from build123d import *

# Parameters (mm, degrees)
SKETCH1_W                = 84.074
SKETCH1_H                = 77.724
BOSS_EXTRUDE1_DEPTH      = 5.08
BOSS_EXTRUDE1_DEPTH_BACK = 5.08
SKETCH2_W                = 84.074
SKETCH2_H                = 77.724
BOSS_EXTRUDE2_DEPTH      = 5.08
BOSS_EXTRUDE2_DEPTH_BACK = 10.16
SKETCH3_W                = 53.086
SKETCH3_H                = 5.08
CUT_EXTRUDE1_DEPTH       = 6.08
CUT_EXTRUDE1_DEPTH_BACK  = 11.16
SKETCH4_W                = 75.946
SKETCH4_H                = 5.08
CUT_EXTRUDE2_DEPTH       = 6.08
CUT_EXTRUDE2_DEPTH_BACK  = 11.16
SKETCH5_W                = 75.946
SKETCH5_H                = 7.62
BOSS_EXTRUDE3_DEPTH      = 5.08
BOSS_EXTRUDE3_DEPTH_BACK = 10.16
SKETCH10_R               = 5.08
CUT_EXTRUDE4_DEPTH       = 6.08
CUT_EXTRUDE4_DEPTH_BACK  = 11.16
FILLET1_R                = 10.16
SKETCH14_W               = 63.5
SKETCH14_H               = 3.429
BOSS_EXTRUDE7_DEPTH      = 3.048
CUT_EXTRUDE6_START       = -16.24
SKETCH15_R               = 2.54
SKETCH15_W               = 7.62
SKETCH15_H               = 3.048
CUT_EXTRUDE6_DEPTH       = 20.288
SKETCH7_W                = 34.036
SKETCH7_H                = 5.08
CUT_EXTRUDE7_DEPTH       = 5.064


with BuildPart() as part:
    # Sketch1 → Boss-Extrude1 (new body, two sides)
    with BuildSketch(Plane(origin=(0, 0, 0), x_dir=(1, 0, 0), z_dir=(0, 1, 0))) as boss_extrude1_sk:
        Rectangle(SKETCH1_W, SKETCH1_H)
    extrude(amount=BOSS_EXTRUDE1_DEPTH)
    extrude(boss_extrude1_sk.sketch, amount=-BOSS_EXTRUDE1_DEPTH_BACK)

    # Sketch2 → Boss-Extrude2 (add, two sides)
    with BuildSketch(Plane(origin=(0, 5.08, 0), x_dir=(1, 0, 0), z_dir=(0, 1, 0))) as boss_extrude2_sk:
        Rectangle(SKETCH2_W, SKETCH2_H)
        Polygon((-37.973, -29.718), (-37.973, 29.718), (-25.273, 29.718), (-25.273, 34.798), (27.813, 34.798), (27.813, 29.718), (37.973, 29.718), (37.973, -29.718), (27.813, -29.718), (27.813, -34.798), (-25.273, -34.798), (-25.273, -29.718), align=None, mode=Mode.SUBTRACT)
    extrude(amount=BOSS_EXTRUDE2_DEPTH)
    extrude(boss_extrude2_sk.sketch, amount=-BOSS_EXTRUDE2_DEPTH_BACK)

    # Sketch3 → Cut-Extrude1 (cut, two sides)
    with BuildSketch(Plane(origin=(0, 5.08, 0), x_dir=(1, 0, 0), z_dir=(0, 1, 0))) as cut_extrude1_sk:
        with Locations((1.27, 32.258)):
            Rectangle(SKETCH3_W, SKETCH3_H)
        with Locations((1.27, -32.258)):
            Rectangle(SKETCH3_W, SKETCH3_H)
    extrude(amount=CUT_EXTRUDE1_DEPTH, mode=Mode.SUBTRACT)
    extrude(cut_extrude1_sk.sketch, amount=-CUT_EXTRUDE1_DEPTH_BACK, mode=Mode.SUBTRACT)

    # Sketch4 → Cut-Extrude2 (cut, two sides)
    with BuildSketch(Plane(origin=(0, 5.08, 0), x_dir=(1, 0, 0), z_dir=(0, 1, 0))) as cut_extrude2_sk:
        with Locations((0, 27.178)):
            Rectangle(SKETCH4_W, SKETCH4_H)
        with Locations((0, -27.178)):
            Rectangle(SKETCH4_W, SKETCH4_H)
    extrude(amount=CUT_EXTRUDE2_DEPTH, mode=Mode.SUBTRACT)
    extrude(cut_extrude2_sk.sketch, amount=-CUT_EXTRUDE2_DEPTH_BACK, mode=Mode.SUBTRACT)

    # Sketch5 → Boss-Extrude3 (add, two sides)
    with BuildSketch(Plane(origin=(0, 5.08, 0), x_dir=(1, 0, 0), z_dir=(0, 1, 0))) as boss_extrude3_sk:
        with Locations((0, 20.828)):
            Rectangle(SKETCH5_W, SKETCH5_H)
        with Locations((0, -20.828)):
            Rectangle(SKETCH5_W, SKETCH5_H)
    extrude(amount=BOSS_EXTRUDE3_DEPTH)
    extrude(boss_extrude3_sk.sketch, amount=-BOSS_EXTRUDE3_DEPTH_BACK)

    # Sketch10 → Cut-Extrude4 (cut, two sides)
    with BuildSketch(Plane(origin=(0, 5.08, 0), x_dir=(1, 0, 0), z_dir=(0, 1, 0))) as cut_extrude4_sk:
        with Locations((3.937, 0)):
            Circle(SKETCH10_R)
    extrude(amount=CUT_EXTRUDE4_DEPTH, mode=Mode.SUBTRACT)
    extrude(cut_extrude4_sk.sketch, amount=-CUT_EXTRUDE4_DEPTH_BACK, mode=Mode.SUBTRACT)

    # Fillet1
    fillet1_edges = [part.edges().sort_by_distance(p)[0] for p in [
        (42.037, 2.54, 38.862),
        (-42.037, 2.54, 38.862),
        (-42.037, 2.54, -38.862),
        (42.037, 2.54, -38.862),
    ]]
    fillet(fillet1_edges, radius=FILLET1_R)

    # Sketch14 → Boss-Extrude7 (add)
    with BuildSketch(Plane(origin=(0, 10.16, 0), x_dir=(1, 0, 0), z_dir=(0, 1, 0))):
        with Locations((1.015527002, -20.828)):
            Rectangle(SKETCH14_W, SKETCH14_H)
        with Locations((0.914410511, 20.828)):
            Rectangle(SKETCH14_W, SKETCH14_H)
    extrude(amount=BOSS_EXTRUDE7_DEPTH)

    # Sketch15 → Cut-Extrude6 (cut)
    with BuildSketch(Plane(origin=(0, 10.16, 0), x_dir=(1, 0, 0), z_dir=(0, 1, 0)).offset(CUT_EXTRUDE6_START)):
        with Locations((32.893, 34.29)):
            Circle(SKETCH15_R)
        with Locations((-31.877, 33.782)):
            Rectangle(SKETCH15_W, SKETCH15_H)
    cut_extrude6 = extrude(amount=CUT_EXTRUDE6_DEPTH, mode=Mode.SUBTRACT)

    # Mirror1: Cut-Extrude6 across plane
    add(cut_extrude6.mirror(Plane.XY), mode=Mode.SUBTRACT)

    # Sketch7 → Cut-Extrude7 (cut, through all)
    with BuildSketch(Plane.ZY.offset(-37.973)):
        with Locations((0, 7.62)):
            Rectangle(SKETCH7_W, SKETCH7_H)
    extrude(amount=-CUT_EXTRUDE7_DEPTH, mode=Mode.SUBTRACT)


solid = part.part
Check sheet for the modelled part. Datum: model origin and axes. Units: mm. A direction names the side the tool comes from. Round coordinates to 2 decimals unless told otherwise and drop trailing zeros. Write each loop counter-clockwise with the first axis right and the second up, starting at its lowest first coordinate (ties: lowest second). Pieces come first, ordered by that corner, then holes. Notation, with made-up numbers: (76, 54) -> (111, 54) arc R35 cw to (111, 88) -> close; hole circle Ø8 at (7.25, -23). An arc over 180 degrees is marked (long way). Answer as CSV lines item,"result". Start each with the question number.
1) Section check C-C on x = -34. Enter the section's corners in (y, z).
2) Release check for a two-part mould opening along Z. For faces 1 (the cylindrical face through (34.26, 2.43, 36.43)), 2 (the cylindrical face through (-39.14, 2.433, -35.807)), 3 (the flat face through (-42.037, 2, 0)) record: pulls with the +Z half, pulls with the -Z half, needs draft (parallel to the pull), parting line crosses it, or undercut.
3) Material ranges on line 1 (Z direction, x = 17, y = 8.25); line 2 (Z direction, x = -20, y = 2.25); line 3 (Z direction, x = -36, y = -0.5), recorded low to high. Write a range as from..to.
4) Tool access check on faces 4 (the flat face through (-37.973, 2, -27)), 5 (the flat face through (1, 8, 17.018)), 6 (the flat face through (0, 12, -19.114)), 7 (the flat face through (0, 12, -22.542)). Record the directions out of +Z, -Z, +X, -X, +Y, -Y that give a thin tool (end or side, any length) a straight path to the whole face; none if there is none.
5) Section check A-A on x = 29. Enter the section's corners in (y, z), and give its area (3 significant figures).
6) Section check D-D on y = 6.75. State how many separate pieces and enclosed holes the cut face has, and give its area (3 significant figures).
7) Go/stop test with flat-tipped pins: P1, Ø6, axis at x = 32.893, z = -34.29, coming from the -Y side; P2, Ø3.5, axis at y = 3, z = -34.5, coming from the -X side; P3, Ø1.5, axis at y = 12.5, z = 20.5, coming from the +X side; P4, Ø3.5, axis at y = 5, z = 34, coming from the -X side. Record where each tip stops, or that it passes through.
8) Section check B-B on z = 0. Enter the section's corners in (x, y), and give its area (3 significant figures).
Found:
1,outline,"(-5.08, -38.64) -> (10.16, -38.64) -> (10.16, -35.31) -> (-5.08, -35.31) -> close; (-5.08, -32.26) -> (10.16, -32.26) -> (10.16, -29.72) -> (-5.08, -29.72) -> close; (-5.08, -24.64) -> (10.16, -24.64) -> (10.16, -17.02) -> (5.08, -17.02) -> (5.08, 17.02) -> (10.16, 17.02) -> (10.16, 24.64) -> (-5.08, 24.64) -> close; (-5.08, 29.72) -> (10.16, 29.72) -> (10.16, 32.26) -> (-5.08, 32.26) -> close; (-5.08, 35.31) -> (10.16, 35.31) -> (10.16, 38.64) -> (-5.08, 38.64) -> close"
2,face 1,"undercut"
2,face 2,"pulls with the -Z half"
2,face 3,"needs draft"
3,line 1,"z = -38.86..-34.8, -24.64..-17.02, 17.02..24.64, 34.8..38.86"
3,line 2,"z = -38.86..-34.8, -24.64..24.64, 34.8..38.86"
3,line 3,"z = -37.99..-29.72, -24.64..24.64, 29.72..37.99"
4,face 4,"+Y, -Y"
4,face 5,"+X, +Y"
4,face 6,"+X, -X, +Y"
4,face 7,"-Z, +X, -X, +Y"
5,outline,"(-5.08, -38.86) -> (10.16, -38.86) -> (10.16, -29.72) -> (-5.08, -29.72) -> close; (-5.08, -24.64) -> (10.16, -24.64) -> (10.16, -22.54) -> (13.21, -22.54) -> (13.21, -19.11) -> (10.16, -19.11) -> (10.16, -17.02) -> (5.08, -17.02) -> (5.08, 17.02) -> (10.16, 17.02) -> (10.16, 19.11) -> (13.21, 19.11) -> (13.21, 22.54) -> (10.16, 22.54) -> (10.16, 24.64) -> (-5.08, 24.64) -> close; (-5.08, 29.72) -> (10.16, 29.72) -> (10.16, 38.86) -> (-5.08, 38.86) -> close"
5,area,"878 mm^2"
6,separate pieces,"1"
6,enclosed holes,"6"
6,area,"2,320 mm^2"
7,P1,"stops at y = -5.08"
7,P2,"stops at x = -41.2"
7,P3,"stops at x = 32.77"
7,P4,"stops at x = -41.4"
8,outline,"(-42.04, -5.08) -> (-1.14, -5.08) -> (-1.14, 5.08) -> (-37.97, 5.08) -> (-37.97, 10.16) -> (-42.04, 10.16) -> close; (9.02, -5.08) -> (42.04, -5.08) -> (42.04, 5.08) -> (9.02, 5.08) -> close"
8,area,"772 mm^2"
